Input: part model. Units: mm. Frame: model coordinates. Face numbers are marked on the shaded views. A direction names the side the tool comes from. Round coordinates to 2 decimals unless told otherwise and drop trailing zeros. Loops run counter-clockwise (first coordinate to the right, second up) from the corner with the lowest first, then second, coordinate; pieces in that order, holes last.
1) Access query for the marked faces 1, 2 and 3. Directions: +Z, -Z, +X, -X, +Y, -Y. A direction counts if a zero-diameter tool reaches every point of the face in a straight line with its end or side. Return the directions, or none.
2) First-contact query: pin 1 (5 mm diameter, centred on y = -157.5, z = 179.5, fed in from -X); pin 2 (2 mm diameter, centred on x = -25.5, y = -170, fed in from +Z); pin 3 (13 mm diameter, centred on x = 18, z = 182.5, fed in from +Y). Flat tips, straight axial feed; report the tip coordinate or a pass-through.
3) Section C-C, the plane z = 22.5. Return loops of the section in (x, y).
4) Section B-B, the plane x = -20. Return loops of the section in (y, z), and give its area (3 significant figures).
5) Ray query, line 1 along X through (y, z) = (-195.5, 63.5); line 2 along Y through (x, z) = (44.5, 64); line 3 along Z through (x, y) = (-61.5, -53). Return the intervals inside material, ascending.
6) Section A-A, the plane y = -86.5. Return loops of the section in (x, z), and give its area (3 significant figures).
7) Section D-D, the plane z = 114. Return loops of the section in (x, y), and give its area (3 significant figures).
8) Draft query along Z for the marked faces 4, 5 and 6. Return one class per face: pulls with the +Z half, pulls with the -Z half, needs draft (parallel to the pull), parting line crosses it, or undercut.
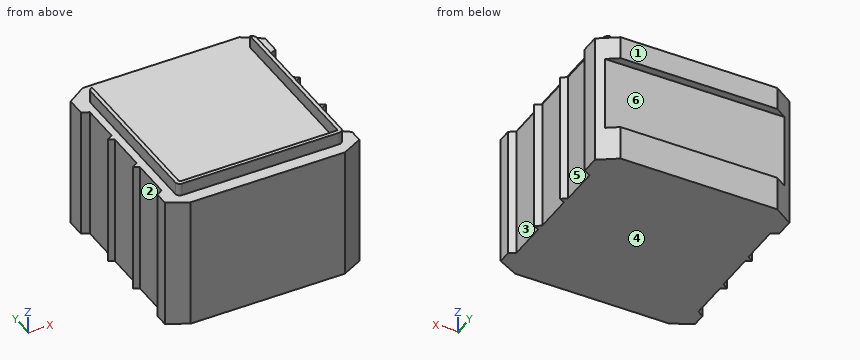
from build123d import *

# Parameters (mm, degrees)
BOSS_EXTRUDE1_DEPTH = 173.478
BOSS_EXTRUDE2_DEPTH = 16.522
SKETCH5_W           = 256
SKETCH5_H           = 98.478
CUT_EXTRUDE3_DEPTH  = 10


with BuildPart() as part:
    # Sketch1 → Boss-Extrude1 (new body)
    with BuildSketch(Plane.XY):
        Polygon((-103.1895488, 0), (103.1895488, 0), (128, -16.432610434), (128, -40.962966098), (118.774155672, -45.61934731), (118.774155672, -97.61934731), (126.583328469, -102.791566604), (119.25400561, -106.490753372), (119.25400561, -158.490753372), (127.063178407, -163.662972666), (119.733855548, -167.362159434), (119.733855548, -219.362159434), (128, -224.837043001), (128, -242.345271931), (101.558790198, -256), (-101.558790198, -256), (-128, -242.345271931), (-128, -224.837043001), (-119.733855548, -219.362159434), (-119.733855548, -167.362159434), (-127.063178407, -163.662972666), (-119.25400561, -158.490753372), (-119.25400561, -106.490753372), (-126.583328469, -102.791566604), (-118.774155672, -97.61934731), (-118.774155672, -45.61934731), (-128, -40.962966098), (-128, -16.432610434), align=None)
    extrude(amount=BOSS_EXTRUDE1_DEPTH)

    # Sketch3 → Boss-Extrude2 (add)
    with BuildSketch(Plane.XY.offset(173.478)):
        with BuildLine():
            Line((-109.25400561, -30.77642723), (-109.25400561, -233.134965715))
            ThreePointArc((-109.25400561, -233.134965715), (-107.53617684, -237.28217123), (-103.388971325, -239))
            Line((-103.388971325, -239), (103.388971325, -239))
            ThreePointArc((103.388971325, -239), (107.53617684, -237.28217123), (109.25400561, -233.134965715))
            Line((109.25400561, -233.134965715), (109.25400561, -32.174007784))
            ThreePointArc((109.25400561, -32.174007784), (108.447882002, -27.049094521), (104.25400561, -23.99524907))
            Line((104.25400561, -23.99524907), (104.25400561, -231.784495248))
            ThreePointArc((104.25400561, -231.784495248), (104.136715259, -232.916299233), (103.789829206, -234))
            Line((103.789829206, -234), (-101.829987525, -234))
            ThreePointArc((-101.829987525, -234), (-103.544027151, -233.290021541), (-104.25400561, -231.575981915))
            Line((-104.25400561, -231.575981915), (-104.25400561, -23.99524907))
            ThreePointArc((-104.25400561, -23.99524907), (-107.868861491, -26.563815889), (-109.25400561, -30.77642723))
        make_face()
    extrude(amount=BOSS_EXTRUDE2_DEPTH)

    # Sketch5 → Cut-Extrude3 (cut)
    with BuildSketch(Plane(origin=(0, 0, 0), x_dir=(1, 0, 0), z_dir=(0, 1, 0))):
        with Locations((0, -94.239)):
            Rectangle(SKETCH5_W, SKETCH5_H)
    extrude(amount=-CUT_EXTRUDE3_DEPTH, mode=Mode.SUBTRACT)


solid = part.part
Final values:
1. face 1: +Z, -Z, +X, -X, +Y
1. face 2: +Z, -Z, -X
1. face 3: +Z, -Z, +X
2. pin 1: stops at x = -109.25
2. pin 2: stops at z = 173.48
2. pin 3: stops at y = -234
3. outline: (-128, -242.35) - (-101.56, -256) - (101.56, -256) - (128, -242.35) - (128, -224.84) - (119.73, -219.36) - (119.73, -167.36) - (127.06, -163.66) - (119.25, -158.49) - (119.25, -106.49) - (126.58, -102.79) - (118.77, -97.62) - (118.77, -45.62) - (128, -40.96) - (128, -16.43) - (103.19, 0) - (-103.19, 0) - (-128, -16.43) - (-128, -40.96) - (-118.77, -45.62) - (-118.77, -97.62) - (-126.58, -102.79) - (-119.25, -106.49) - (-119.25, -158.49) - (-127.06, -163.66) - (-119.73, -167.36) - (-119.73, -219.36) - (-128, -224.84) - close
4. outline: (-256, 0) - (0, 0) - (0, 45) - (-10, 45) - (-10, 143.48) - (0, 143.48) - (0, 173.48) - (-234, 173.48) - (-234, 190) - (-239, 190) - (-239, 173.48) - (-256, 173.48) - close
4. area: 43,500 mm2
5. line 1: x = -119.73 to 119.73
5. line 2: y = -256 to -10
5. line 3: z = 0 to 173.48
6. outline: (-118.77, 0) - (118.77, 0) - (118.77, 173.48) - (109.25, 173.48) - (109.25, 190) - (104.25, 190) - (104.25, 173.48) - (-104.25, 173.48) - (-104.25, 190) - (-109.25, 190) - (-109.25, 173.48) - (-118.77, 173.48) - close
6. area: 41,400 mm2
7. outline: (-128, -242.35) - (-101.56, -256) - (101.56, -256) - (128, -242.35) - (128, -224.84) - (119.73, -219.36) - (119.73, -167.36) - (127.06, -163.66) - (119.25, -158.49) - (119.25, -106.49) - (126.58, -102.79) - (118.77, -97.62) - (118.77, -45.62) - (128, -40.96) - (128, -16.43) - (118.29, -10) - (-118.29, -10) - (-128, -16.43) - (-128, -40.96) - (-118.77, -45.62) - (-118.77, -97.62) - (-126.58, -102.79) - (-119.25, -106.49) - (-119.25, -158.49) - (-127.06, -163.66) - (-119.73, -167.36) - (-119.73, -219.36) - (-128, -224.84) - close
7. area: 59,600 mm2
8. face 4: pulls with the -Z half
8. face 5: needs draft
8. face 6: undercut
